Answer from the drawing. Dimensions are ordinates in mm from the lowest x, y and z of the part. A direction names the side the tool comes from. Give positions to 0.01 mm unless a question says otherwise; leave off trailing zeros. Loops run counter-clockwise (first coordinate to the right, second up) from the corner with the lowest first, then second, coordinate; pieces in that order, holes last. Notation, with made-up numbers: (73.5, 73) -> (92.5, 73) arc R19 ccw to (92.5, 90) -> close; hole circle Ø6 at (-18.75, -7). An arc over 180 degrees is marked (long way). Return JSON: item names as keys, results as strings. Group by question number.
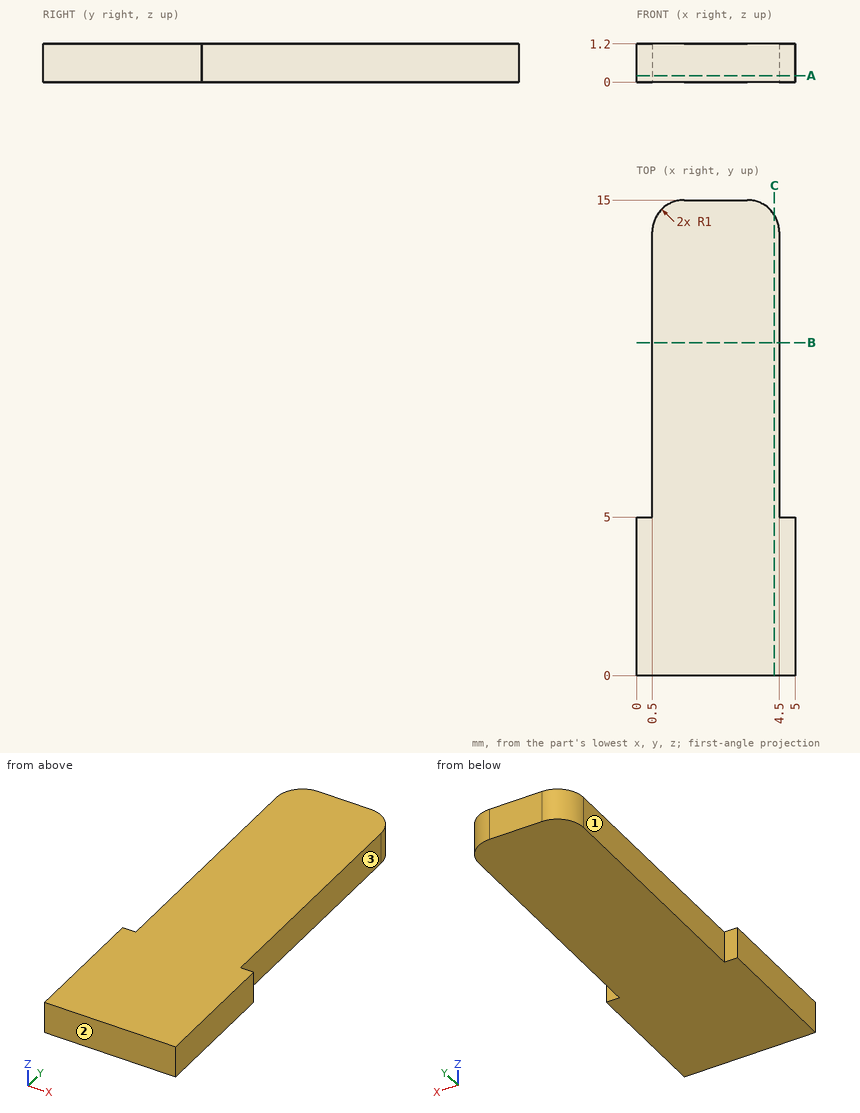
1. Section B-B on y = 10.5 is taken. Determine the outline of the cut face in (x, z), then the cut area to 3 significant figures.
2. Flat-ended cylindrical pins translate along their axes: pin 1 Ø1 at (x, y) = (1.5, 8.5) entering from -Z; pin 2 Ø0.6 at (x, z) = (0, 0.5) entering from +Y. Find the tip coordinate at first contact, or state that the pin passes through.
3. Section C-C on x = 4.35 is taken. Determine the outline of the cut face in (y, z).
4. Straight lines are drawn through the part: line 1 (X direction, y = 11.75, z = 0.95); line 2 (Y direction, x = 1.45, z = 0.95); line 3 (Y direction, x = 4.7, z = 0.9). For each, find the intervals that lie inside material, in ascending order. Write a range as from..to.
5. Which of the six approach directions +Z, -Z, +X, -X, +Y, -Y give full straight-line access (tool end or side, diameter ignored) to the marked faces 1, 2 and 3?
6. Section A-A on z = 0.2 is taken. Determine the outline of the cut face in (x, y), then the cut area to 3 significant figures.
Completed:
{
 "1": {"outline": "(0.5, 0) -> (4.5, 0) -> (4.5, 1.2) -> (0.5, 1.2) -> close", "area": "4.80 mm²"},
 "2": {"pin 1": "stops at z = 0", "pin 2": "stops at y = 5"},
 "3": {"outline": "(0, 0) -> (14.53, 0) -> (14.53, 1.2) -> (0, 1.2) -> close"},
 "4": {"line 1": "x = 0.5..4.5", "line 2": "y = 0..15", "line 3": "y = 0..5"},
 "5": {"face 1": "+Z, -Z, -X, +Y", "face 2": "+Z, -Z, +X, -X, -Y", "face 3": "+Z, -Z, +X, +Y"},
 "6": {"outline": "(0, 0) -> (5, 0) -> (5, 5) -> (4.5, 5) -> (4.5, 14) arc R1 ccw to (3.5, 15) -> (1.5, 15) arc R1 ccw to (0.5, 14) -> (0.5, 5) -> (0, 5) -> close", "area": "64.6 mm²"}
}
